Verification items for the finished model (mm, model axes). Face numbers are marked on the shaded views. A direction names the side the tool comes from. Round coordinates to 2 decimals unless told otherwise and drop trailing zeros. Write each loop counter-clockwise with the first axis right and the second up, starting at its lowest first coordinate (ties: lowest second). Pieces come first, ordered by that corner, then holes. Notation, with made-up numbers: M 9.5,0.5 L 39.5,0.5 A21 cw 39.5,16.5 Z; hole C -26,39 d10. An arc over 180 degrees is marked long. Write each question's results on one line, items separated by ' | '.
from build123d import *

# Parameters (mm, degrees)
SKETCH_1_R          = 1.5
SKETCH_1_W          = 5
SKETCH_1_H          = 5
SKETCH_1_R_2        = 2
EXTRUDE_1_DEPTH     = 2
SKETCH_1_3_R        = 2
EXTRUDE_2_DEPTH     = 34
EXTRUDE_START       = 4
SKETCH_2_R          = 17.5
EXTRUDE_3_DEPTH     = 25
CHAMFER_1_SIZE      = 3
CUT_EXTRUDE_1_DEPTH = 25
CHAMFER_2_SIZE      = 0.5


with BuildPart() as part:
    # Sketch 1 → Extrude 1 (new body)
    # profile 1 of 6: a face of its own
    with BuildSketch(Plane(origin=(0, 0, 0), x_dir=(1, 0, 0), z_dir=(0, 1, 0))):
        with BuildLine():
            Line((-12.5, -2.5), (-2.5, -2.5))
            Line((-2.5, -2.5), (-2.5, 2.5))
            Line((-2.5, 2.5), (-12.5, 2.5))
            ThreePointArc((-12.5, 2.5), (-15, 0), (-12.5, -2.5))
        make_face()
        with Locations(Location((-12.5, 0, 0), (0, 0, 270))):
            Circle(SKETCH_1_R, mode=Mode.SUBTRACT)
        with Locations(Location((-8, 0, 0), (0, 0, 270))):
            Circle(SKETCH_1_R, mode=Mode.SUBTRACT)
    # profile 2 of 6: a face of its own
    with BuildSketch(Plane(origin=(0, 0, 0), x_dir=(1, 0, 0), z_dir=(0, 1, 0))):
        Rectangle(SKETCH_1_W, SKETCH_1_H)
        Circle(SKETCH_1_R_2, mode=Mode.SUBTRACT)
    # profile 3 of 6: a face of its own
    with BuildSketch(Plane(origin=(0, 0, 0), x_dir=(1, 0, 0), z_dir=(0, 1, 0))):
        Circle(SKETCH_1_R_2)
    # profile 4 of 6: a face of its own
    with BuildSketch(Plane(origin=(0, 0, 0), x_dir=(1, 0, 0), z_dir=(0, 1, 0))):
        with BuildLine():
            Line((-2.5, -2.5), (-2.5, -9.5))
            ThreePointArc((-2.5, -9.5), (0, -12), (2.5, -9.5))
            Line((2.5, -9.5), (2.5, -2.5))
            Line((2.5, -2.5), (-2.5, -2.5))
        make_face()
        with Locations(Location((0, -9.5, 0), (0, 0, 270))):
            Circle(SKETCH_1_R, mode=Mode.SUBTRACT)
    # profile 5 of 6: a face of its own
    with BuildSketch(Plane(origin=(0, 0, 0), x_dir=(1, 0, 0), z_dir=(0, 1, 0))):
        with BuildLine():
            Line((-2.5, 9.5), (-2.5, 2.5))
            Line((-2.5, 2.5), (2.5, 2.5))
            Line((2.5, 2.5), (2.5, 9.5))
            ThreePointArc((2.5, 9.5), (0, 12), (-2.5, 9.5))
        make_face()
        with Locations(Location((0, 9.5, 0), (0, 0, 270))):
            Circle(SKETCH_1_R, mode=Mode.SUBTRACT)
    # profile 6 of 6: a face of its own
    with BuildSketch(Plane(origin=(0, 0, 0), x_dir=(1, 0, 0), z_dir=(0, 1, 0))):
        with BuildLine():
            Line((2.5, 2.5), (2.5, -2.5))
            Line((2.5, -2.5), (12.5, -2.5))
            ThreePointArc((12.5, -2.5), (15, 0), (12.5, 2.5))
            Line((12.5, 2.5), (2.5, 2.5))
        make_face()
        with Locations(Location((8, 0, 0), (0, 0, 270))):
            Circle(SKETCH_1_R, mode=Mode.SUBTRACT)
        with Locations(Location((12.5, 0, 0), (0, 0, 270))):
            Circle(SKETCH_1_R, mode=Mode.SUBTRACT)
    extrude(amount=-EXTRUDE_1_DEPTH)

    # Sketch 1_3 → Extrude 2 (add)
    with BuildSketch(Plane(origin=(0, 0, 0), x_dir=(1, 0, 0), z_dir=(0, 1, 0))):
        with Locations(Location((0, 0, 0), (0, 0, 270))):
            Circle(SKETCH_1_3_R)
    extrude(amount=EXTRUDE_2_DEPTH)

    # Sketch 2 → Extrude 3 (add)
    with BuildSketch(Plane(origin=(0, 0, 0), x_dir=(1, 0, 0), z_dir=(0, 1, 0)).offset(EXTRUDE_START)):
        with Locations(Location((0, 0, 0), (0, 0, 270))):
            Circle(SKETCH_2_R)
    extrude(amount=EXTRUDE_3_DEPTH)

    # Chamfer 1
    chamfer_1_edges = [part.edges().sort_by_distance(p)[0] for p in [
        (0, 29, -17.5),
    ]]
    chamfer(chamfer_1_edges, length=CHAMFER_1_SIZE)

    # Sketch 4 → Cut-Extrude 1 (cut)
    with BuildSketch(Plane(origin=(0, 29, 0), x_dir=(1, 0, 0), z_dir=(0, 1, 0))):
        with BuildLine():
            Line((-1, 11.456439237), (-1, 4.898979486))
            ThreePointArc((-1, 4.898979486), (-3.535533906, 3.535533906), (-4.898979486, 1))
            Line((-4.898979486, 1), (-11.456439237, 1))
            ThreePointArc((-11.456439237, 1), (-8.131727984, 8.131727984), (-1, 11.456439237))
        make_face()
        with BuildLine():
            Line((-11.456439237, -1), (-4.898979486, -1))
            ThreePointArc((-4.898979486, -1), (-3.535533906, -3.535533906), (-1, -4.898979486))
            Line((-1, -4.898979486), (-1, -11.456439237))
            ThreePointArc((-1, -11.456439237), (-8.131727984, -8.131727984), (-11.456439237, -1))
        make_face()
        with BuildLine():
            Line((11.456439237, 1), (4.898979486, 1))
            ThreePointArc((4.898979486, 1), (3.535533906, 3.535533906), (1, 4.898979486))
            Line((1, 4.898979486), (1, 11.456439237))
            ThreePointArc((1, 11.456439237), (8.131727984, 8.131727984), (11.456439237, 1))
        make_face()
        with BuildLine():
            Line((1, -11.456439237), (1, -4.898979486))
            ThreePointArc((1, -4.898979486), (3.535533906, -3.535533906), (4.898979486, -1))
            Line((4.898979486, -1), (11.456439237, -1))
            ThreePointArc((11.456439237, -1), (8.131727984, -8.131727984), (1, -11.456439237))
        make_face()
    extrude(amount=-CUT_EXTRUDE_1_DEPTH, mode=Mode.SUBTRACT)

    # Chamfer 2
    chamfer_2_edges = [part.edges().sort_by_distance(p)[0] for p in [
        (0, 34, -2),
    ]]
    chamfer(chamfer_2_edges, length=CHAMFER_2_SIZE)


solid = part.part
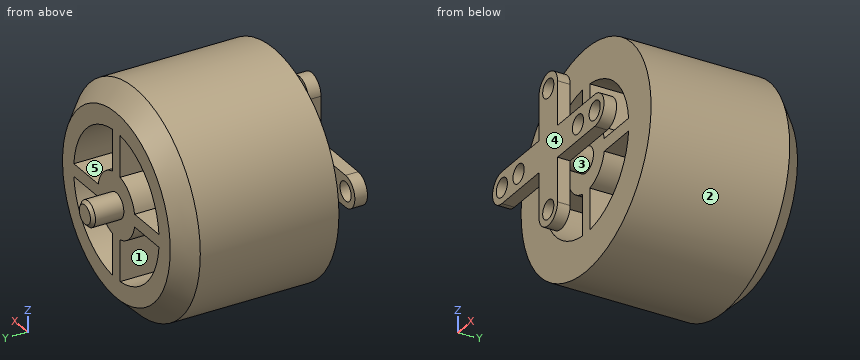
1) Material ranges on line 1 (X direction, y = -1, z = 0); line 2 (X direction, y = 4.5, z = 6.5); line 3 (X direction, y = 6, z = 8), recorded low to high. Write a range as [from, to].
Calculated:
line 1: x = [-15, -14], [-11, -9.5], [-6.5, 6.5], [9.5, 11], [14, 15] | line 2: x = [-16.25, -9.49], [-1, 1], [9.49, 16.25] | line 3: x = [-15.56, -8.26], [-1, 1], [8.26, 15.56]
2) Sectioned sample at D-D, the plane y = 22. Record the cut outline in (x, z), and give its area (3 significant figures).
Calculated:
outline: C 0,0 d35; hole M -11.46,-1 A11.5 ccw -1,-11.46 L -1,-4.9 A5 cw -4.9,-1 Z; hole M -11.46,1 L -4.9,1 A5 cw -1,4.9 L -1,11.46 A11.5 ccw Z; hole M 1,-11.46 A11.5 ccw 11.46,-1 L 4.9,-1 A5 cw 1,-4.9 Z; hole M 1,4.9 A5 cw 4.9,1 L 11.46,1 A11.5 ccw 1,11.46 Z | area: 677 mm²
3) Sectioned sample at A-A, the plane y = 27. Record the cut outline in (x, z), and give its area (3 significant figures).
Calculated:
outline: C 0,0 d33; hole M -11.46,-1 A11.5 ccw -1,-11.46 L -1,-4.9 A5 cw -4.9,-1 Z; hole M -11.46,1 L -4.9,1 A5 cw -1,4.9 L -1,11.46 A11.5 ccw Z; hole M 1,-11.46 A11.5 ccw 11.46,-1 L 4.9,-1 A5 cw 1,-4.9 Z; hole M 1,4.9 A5 cw 4.9,1 L 11.46,1 A11.5 ccw 1,11.46 Z | area: 571 mm²
4) Access from +Z, -Z, +X, -X, +Y, -Y to the whole of each face (thin tool, end or side, straight path). Record for the marked faces 1 and 2.
Calculated:
face 1: +Y | face 2: +Y, -Y
5) Draft check along Z on the marked faces 3, 4 and 5. Enter one of: pulls with the +Z half, pulls with the -Z half, needs draft (parallel to the pull), parting line crosses it, or undercut.
Calculated:
face 3: parting line crosses it | face 4: needs draft | face 5: undercut
6) Depth check by flat-ended pin: P1, Ø3, axis at x = -3.5, z = -9.5, coming from the +Y side; P2, Ø1, axis at y = -1, z = -7, coming from the +X side; P3, Ø2.5, axis at x = 0, z = -9.5, coming from the -Y side. Enter the tip coordinate at first touch or a pass-through.
Calculated:
P1: stops at y = 29 | P2: stops at x = 2.5 | P3: stops at y = 4
7) Sectioned sample at B-B, the plane z = 0. Count the separate pieces of the cut face and the enclosed holes in it, and give its area (3 significant figures).
Calculated:
separate pieces: 5 | enclosed holes: 0 | area: 938 mm²
